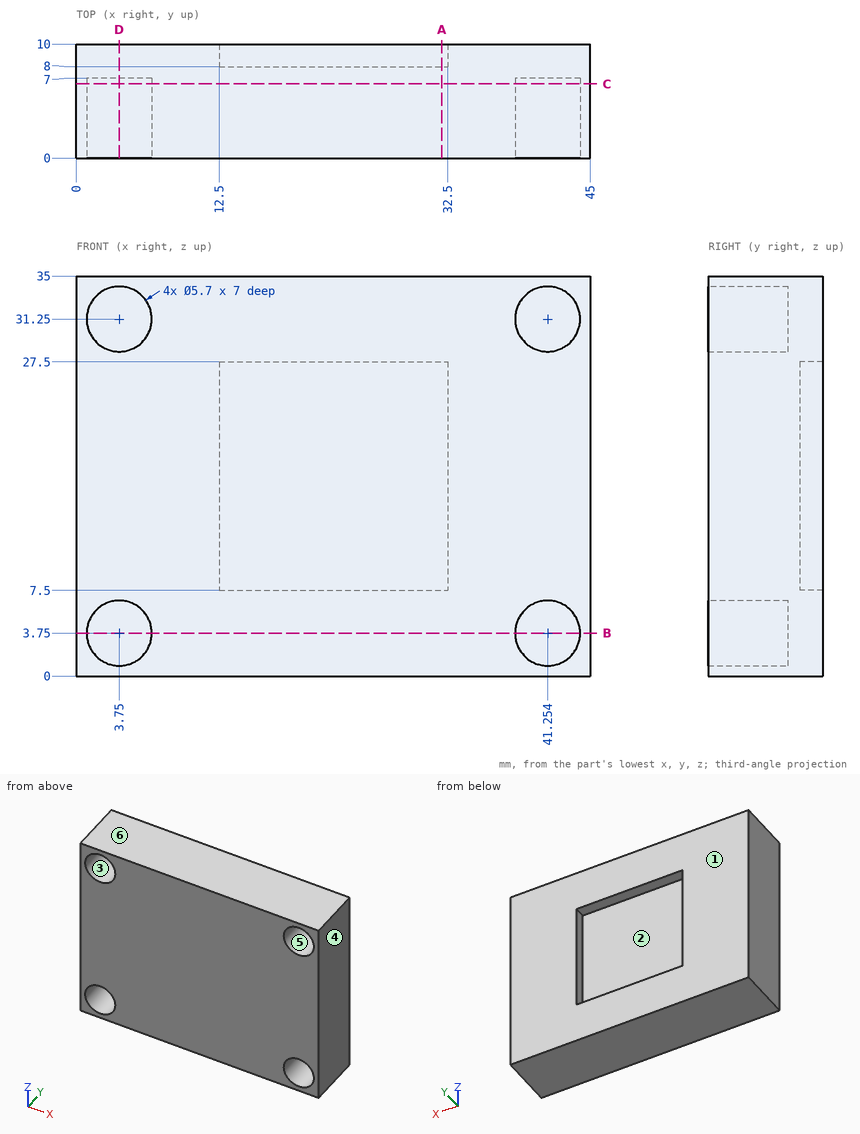
Could you check a few things on this drawing? It's one solid part, dimensions in mm from its lowest x, y, z. A direction names the side the tool comes from. Coordinates: 2 decimals unless noted, no trailing zeros. Loops run counter-clockwise (first coordinate to the right, second up) from the corner with the lowest first, then second, coordinate; pieces in that order, holes last. Notation, with made-up numbers: (37, 29) - (44, 29) arc R23 cw to (44, 67) - close; hole circle Ø8 at (51, 63). An arc over 180 degrees is marked (long way). Answer as a JSON object with one key per item and string values. Group by question number.
Item 1: If we section it at C-C (y = 6.5): State how many separate pieces and enclosed holes the cut face has, plus the area to 3 significant figures.
Item 2: If we mould it in two halves opening along X, with no side actions, what happens to the marked faces 4, 5 and 6? For each: released by +X, released by -X, zero draft, split by the parting line, or undercut.
Item 3: If we section it at D-D (x = 3.75): List the corners of the cut face in (y, z) for me, plus the area to 3 significant figures.
Item 4: If we section it at A-A (x = 32): List the corners of the cut face in (y, z) for me, plus the area to 3 significant figures.
Item 5: If we section it at B-B (z = 3.75): List the corners of the cut face in (x, y) for me (1 decimal).
Item 6: For pin 1 (10 mm diameter, centred on x = 24.5, z = 16.5, fed in from +Y); pin 2 (1.7 mm diameter, centred on x = 41, z = 31.5, fed in from -Y), each with a flat end and sliding along its axis, tell me the tip position at first contact or that it passes through.
Item 7: On a 3-axis mill with a long thin cutter (end or side, diameter ignored), from which of +Z, -Z, +X, -X, +Y, -Y can I reach the whole of each face in a straight line? I mean the marked faces 1, 2 and 3. Say none if no direction works.
Item 8: If I drill on L1, parallel to X at y = 5, z = 31.25 (1 decimal); L2, parallel to Z at x = 41, y = 4.25; L3, parallel to X at y = 2, z = 29.5 (1 decimal), over which ranges is the centre line in solid material (lowest first)? Write a range as from..to.
Returned:
{
 "1": {"separate pieces": "1", "enclosed holes": "4", "area": "1,470 mm²"},
 "2": {"face 4": "released by +X", "face 5": "undercut", "face 6": "zero draft"},
 "3": {"outline": "(0, 0) - (10, 0) - (10, 35) - (0, 35) - (0, 34.1) - (7, 34.1) - (7, 28.4) - (0, 28.4) - (0, 6.6) - (7, 6.6) - (7, 0.9) - (0, 0.9) - close", "area": "270 mm²"},
 "4": {"outline": "(0, 0) - (10, 0) - (10, 7.5) - (8, 7.5) - (8, 27.5) - (10, 27.5) - (10, 35) - (0, 35) - close", "area": "310 mm²"},
 "5": {"outline": "(0, 0) - (0.9, 0) - (0.9, 7) - (6.6, 7) - (6.6, 0) - (38.4, 0) - (38.4, 7) - (44.1, 7) - (44.1, 0) - (45, 0) - (45, 10) - (0, 10) - close"},
 "6": {"pin 1": "stops at y = 8", "pin 2": "stops at y = 7"},
 "7": {"face 1": "+Z, -Z, +X, -X, +Y", "face 2": "+Y", "face 3": "-Y"},
 "8": {"L1": "x = 0..0.9, 6.6..38.4, 44.1..45", "L2": "z = 0..0.91, 6.59..28.41, 34.09..35", "L3": "x = 0..1.5, 6..39, 43.5..45"}
}
